Here's the drawing with two shaded views (mm, measured from the low corner). I have some questions. A direction names the side the tool comes from. Coordinates: 2 decimals unless noted, no trailing zeros. Order: outer loops, then holes, each group sorted by start corner. A loop starts at its lowest first (then second) coordinate and runs counter-clockwise, first axis right, second up. Notation, with made-up numbers: (31, 15.25) - (64, 15.25) arc R19 cw to (64, 44.25) - close; hole circle Ø10 at (61.25, -6). An arc over 180 degrees is marked (long way). Answer as CSV lines item,"result". Start each with the question number.
1. I want a section at D-D, the plane z = 0.4. List the corners of the cut face in (x, y) for me, and give its area (3 significant figures).
2. For pin 1 (5 mm diameter, centred on x = 12, y = 2.5, fed in from -Z); pin 2 (1.5 mm diameter, centred on x = 12.5, z = 1.5, fed in from -Y); pin 3 (1 mm diameter, centred on x = 7, z = 0.5, fed in from +Y), each with a flat end and sliding along its axis, tell me the tip position at first contact or that it passes through.
3. I want a section at A-A, the plane z = 2.3. List the corners of the cut face in (x, y) for me, and give its area (3 significant figures).
4. I want a section at C-C, the plane y = 14.5. List the corners of the cut face in (x, z) for me (3 decimals).
5. I want a section at B-B, the plane x = 4.25. List the corners of the cut face in (y, z) for me (3 decimals), and give its area (3 significant figures).
6. For the marked faces 4 and 5, which set-ups out of +Z, -Z, +X, -X, +Y, -Y let a thin tool reach every point of the face, with its end or its side?
7. Thinking about a two-plate mould opening in X: for the marked faces 1, 2 and 3, which applies, released by +X, released by -X, zero draft, split by the parting line, or undercut?
8. I need wall thicknesses on probe 1 along Y at (x, z) = (6.5, 1.15); probe 2 along Z at (x, y) = (6.75, 5) (3 decimals); probe 3 along X at (y, z) = (22, 1.4). Which ranges of each line are inside material? Lowest first, please.
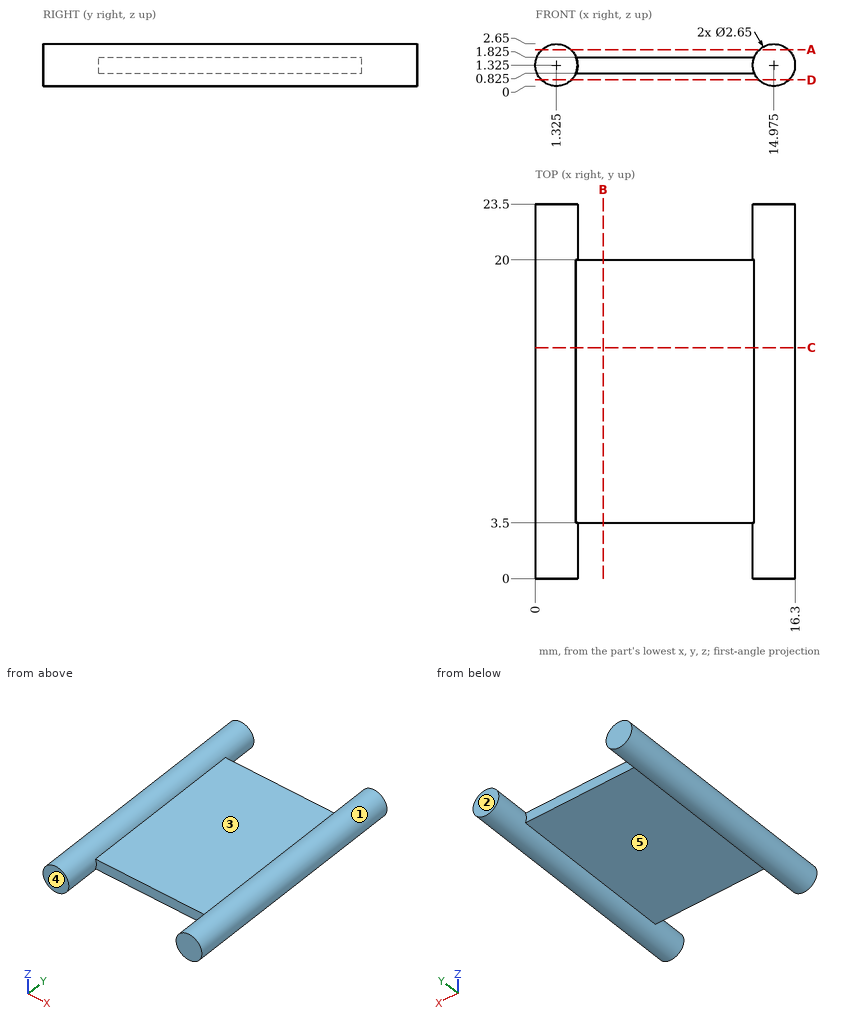
Solved:
1,outline,"(0.38, 0) - (2.27, 0) - (2.27, 23.5) - (0.38, 23.5) - close; (14.03, 0) - (15.92, 0) - (15.92, 23.5) - (14.03, 23.5) - close"
1,area,"89.2 mm2"
2,pin 1,"stops at z = 0.09"
2,pin 2,"stops at y = 3.5"
2,pin 3,"stops at y = 20"
3,outline,"(0.43, 0) - (2.22, 0) - (2.22, 23.5) - (0.43, 23.5) - close; (14.08, 0) - (15.87, 0) - (15.87, 23.5) - (14.08, 23.5) - close"
3,area,"84.3 mm2"
4,outline,"(2.552, 0.825) - (13.748, 0.825) arc R1.325 ccw (long way) to (13.748, 1.825) - (2.552, 1.825) arc R1.325 ccw (long way) to start"
5,outline,"(3.5, 0.825) - (20, 0.825) - (20, 1.825) - (3.5, 1.825) - close"
5,area,"16.5 mm2"
6,face 4,"+Z, -Z, +X, -X, -Y"
6,face 5,"-Z, +Y, -Y"
7,face 1,"undercut"
7,face 2,"zero draft"
7,face 3,"undercut"
8,probe 1,"y = 3.5 to 20"
8,probe 2,"z = 0.825 to 1.825"
8,probe 3,"x = 0 to 2.65, 13.65 to 16.3"
